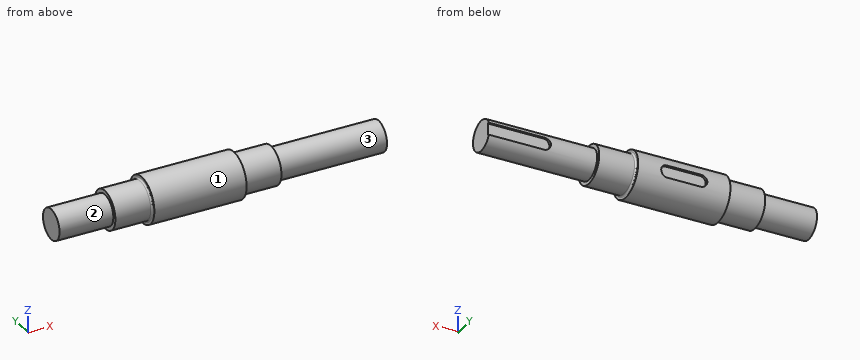
```python
from build123d import *

# Parameters (mm, degrees)
FILLET1_R          = 1
CUT_EXTRUDE1_DEPTH = 2
CUT_EXTRUDE2_DEPTH = 2


with BuildPart() as part:
    # Sketch1 → Revolve2 (revolve)
    with BuildSketch(Plane.XY):
        Polygon((-89, 0), (-89, 10), (-54, 10), (-54, 12.5), (-30, 12.5), (-30, 15), (30, 15), (30, 12.5), (54, 12.5), (54, 10), (89, 10), (124, 10), (124, 0), align=None)
    revolve(axis=Axis((124, 0, 0), (-1, 0, 0)))

    # Fillet1
    fillet1_edges = [part.edges().sort_by_distance(p)[0] for p in [
        (30, -12.5, 0),
        (-30, -12.5, 0),
    ]]
    fillet(fillet1_edges, radius=FILLET1_R)

    # Sketch2 → Cut-Extrude1 (cut)
    with BuildSketch(Plane(origin=(0, 15, 0), x_dir=(1, 0, 0), z_dir=(0, 1, 0))):
        with BuildLine():
            Line((11, -4), (-11, -4))
            ThreePointArc((-11, -4), (-15, 0), (-11, 4))
            Line((-11, 4), (11, 4))
            ThreePointArc((11, 4), (15, 0), (11, -4))
        make_face()
    extrude(amount=-CUT_EXTRUDE1_DEPTH, mode=Mode.SUBTRACT)

    # Sketch3 → Cut-Extrude2 (cut)
    with BuildSketch(Plane(origin=(0, 10, 0), x_dir=(1, 0, 0), z_dir=(0, 1, 0))):
        with BuildLine():
            Line((124, -4), (88, -4))
            ThreePointArc((88, -4), (84, 0), (88, 4))
            Line((88, 4), (124, 4))
            Line((124, 4), (124, -4))
        make_face()
    extrude(amount=-CUT_EXTRUDE2_DEPTH, mode=Mode.SUBTRACT)


solid = part.part
```
Check sheet for the modelled part. Datum: model origin and axes. Units: mm. Face numbers are marked on the shaded views. A direction names the side the tool comes from. Give positions to 0.01 mm unless a question says otherwise; leave off trailing zeros. Loops run counter-clockwise (first coordinate to the right, second up) from the corner with the lowest first, then second, coordinate; pieces in that order, holes last. Notation, with made-up numbers: (83, 20.25) - (88, 20.25) arc R23 cw to (88, 32.25) - close; hole circle Ø10 at (12, 66). An arc over 180 degrees is marked (long way). One line per question, with ' | ' between items. Start each with the question number.
1. Gauge pin test, flat ends, axial feed: pin 1 Ø5 at (x, z) = (14.5, -9) entering from +Y; pin 2 Ø1.5 at (x, z) = (84.5, 12) entering from +Y; pin 3 Ø1 at (x, z) = (33, -6.5) entering from -Y; pin 4 Ø12 at (x, y) = (81.5, -4.5) entering from -Z. Record the tip position at first contact, or that the pin passes through.
2. Cross-section at B-B, the plane y = 0. Enter the section's corners in (x, z), plus the area to 3 significant figures.
3. Cross-section at C-C, the plane x = -50. Enter the section's corners in (y, z).
4. Set-up check for the marked faces 1, 2 and 3: record each of +Z, -Z, +X, -X, +Y, -Y from which the full face is reachable in a straight line by a thin tool's end or side.
5. Material ranges on line 1 along X through (y, z) = (4, -9.5); line 2 along X through (y, z) = (-13, -5); line 3 along Y through (x, z) = (-3.5, -0.5), recorded low to high. Write a range as [from, to].
Check result:
1) pin 1: stops at y = 13.52 | pin 2: passes through | pin 3: stops at y = -10.97 | pin 4: stops at z = -10
2) outline: (-89, -10) - (-54, -10) - (-54, -12.5) - (-31, -12.5) arc R1 cw to (-30, -13.5) - (-30, -15) - (30, -15) - (30, -13.5) arc R1 cw to (31, -12.5) - (54, -12.5) - (54, -10) - (124, -10) - (124, 10) - (54, 10) - (54, 12.5) - (31, 12.5) arc R1 cw to (30, 13.5) - (30, 15) - (-30, 15) - (-30, 13.5) arc R1 cw to (-31, 12.5) - (-54, 12.5) - (-54, 10) - (-89, 10) - close | area: 5,100 mm2
3) outline: circle Ø25 at (0, 0)
4) face 1: +X, -X | face 2: -X | face 3: +X
5) line 1: x = [-54, 54] | line 2: x = [-30, 30] | line 3: y = [-14.99, 13]
